Design review of the part built by this model. Coordinates are the model's own, in mm. A direction names the side the tool comes from. Coordinates: 2 decimals unless noted, no trailing zeros. Order: outer loops, then holes, each group sorted by start corner. A loop starts at its lowest first (then second) coordinate and runs counter-clockwise, first axis right, second up. Notation, with made-up numbers: (-40, -1) -> (18, -1) arc R31 ccw to (18, 32) -> close; hole circle Ø10 at (-29.75, -37). An arc over 180 degrees is marked (long way). Use a Markdown table: item, result. Add a question column.
Q1. The part is to be moulded in two halves that separate along Y. For faces 3 (the face through (-74, -82, 0)), 4 (the face through (110.55, 14.52, 6.59)), 5 (the face through (104.151, 23.128, 5.625)), say which applies: pulls with the +Y half, pulls with the -Y half, needs draft (parallel to the pull), parting line crosses it, or undercut.
Q2. Add section A-A (x = 0). State the section outline as (y, z) points, then the cut area to 3 significant figures.
Q3. Machinability: for faces 1 (the face through (-107.872, 23.954, 11.521)), 2 (the face through (25, 108, 13)), which of the approach directions +Z, -Z, +X, -X, +Y, -Y give a long, thin tool a straight path to every point of the face, cutting with its end or side? Answer none if there is none.
Q4. Wall thickness on probe 1 along X at (y, z) = (0, 12); probe 2 along Y at (x, z) = (42, 1.75); probe 3 along X at (y, z) = (-7.5, 2.25): over which ranges is each line inside the solid? List them lowest first.
Q5. Insertion check: pin 1 (1 mm diameter, centred on x = 88, y = -62.5, fed in from +Z); pin 2 (4 mm diameter, centred on x = 27.5, z = 5, fed in from -Y); pin 3 (3 mm diameter, centred on y = -40.5, z = 7.5, fed in from +X). Each pin has a flat end and moves straight along its axis. Give the tip position at first contact, or say it passes through.
Autodesk Fusion 360 part; units mm, degrees
sketch "Skizze1" plane through (0, 0, 0) normal (1, 0, 0) x (0, 1, 0)
  line L0 (-111.5, 0) -> (-111.5, 10)
  line L1 (-110.5, 10) -> (-109.5, 10)
  line L2 (-111.5, 0) -> (-109.5, 0)
  line L3 (-109.5, 0) -> (-106.5, 6)
  line L4 (-106.5, 6) -> (-109.5, 10)
  line L5 (0, 0) -> (0, 38) construction
  line L6 (-110.5, 10) -> (-110.5, 13)
  line L7 (-110.5, 13) -> (-111.5, 13)
  line L8 (-111.5, 13) -> (-111.5, 10)
  dimension "d2" = 2
  dimension "d3" = 2
  dimension "d4" = 6
  dimension "d5" = 5
  dimension "d6" = 111.5
  dimension "d9" = 3
  dimension "d10" = 1
  dimension "d11" = 10
revolve "Drehen1" add sketch "Skizze1" angle 360 about axis through (0, 0, 0) along (0, 0, 1)
Established:
| question | item | result |
|---|---|---|
| 1 | face 3 | needs draft |
| 1 | face 4 | parting line crosses it |
| 1 | face 5 | undercut |
| 2 | outline | (-111.5, 0) -> (-109.5, 0) -> (-106.5, 6) -> (-109.5, 10) -> (-110.5, 10) -> (-110.5, 13) -> (-111.5, 13) -> close; (106.5, 6) -> (109.5, 0) -> (111.5, 0) -> (111.5, 13) -> (110.5, 13) -> (110.5, 10) -> (109.5, 10) -> close |
| 2 | area | 76.0 mm^2 |
| 3 | face 1 | +Z |
| 3 | face 2 | +Z, +X, -X, +Y, -Y |
| 4 | probe 1 | -111.5 to -110.5, 110.5 to 111.5 |
| 4 | probe 2 | -103.29 to -100.18, 100.18 to 103.29 |
| 4 | probe 3 | -111.25 to -108.12, 108.12 to 111.25 |
| 5 | pin 1 | z = 8.58 |
| 5 | pin 2 | y = -108.54 |
| 5 | pin 3 | x = 104.46 |
